Read the model definition and answer for the solid it produces. Units are mm, in the model's axes. A direction names the side the tool comes from. Coordinates: 2 decimals unless noted, no trailing zeros. Write each loop counter-clockwise with the first axis right and the second up, starting at its lowest first coordinate (ties: lowest second). Pieces come first, ordered by that corner, then holes. Notation, with made-up numbers: (-26, -23) -> (12, -23) arc R16 ccw to (12, -4) -> close; hole circle Ø9 at (-36.75, -19). An arc over 180 degrees is marked (long way). Answer as a JSON object with one key per item and string values. Group by question number.
(1) For a pull along Y with two mould halves and no side action, classify faces 3 (the face through (0, 23, 0)), 4 (the face through (2, 27, 1)), 5 (the face through (0, 0, 0)), 6 (the face through (-2, 28, 0)) as +Y half, -Y half, draft (parallel to the pull), parting line (faces both ways), or undercut.
(2) Find section D-D (z = -1.25). Give the vertices of the cut face in (x, y).
(3) Find section B-B (y = 27). Give the vertices of the cut face in (x, z).
(4) Find section C-C (x = -2.25). Give the vertices of the cut face in (y, z), then the cut area to 3 significant figures.
(5) Which of the six approach directions +Z, -Z, +X, -X, +Y, -Y give full straight-line access (tool end or side, diameter ignored) to faces 1 (the face through (-1.3, 25.8, 0)), 2 (the face through (0, 15, -3))?
(6) Straight lines are drawn through the part: L1, parallel to Y at x = -2.1, z = 0; L2, parallel to Y at x = -1, z = -0.5; L3, parallel to Z at x = -2, y = 27. For each, find the intervals that lie inside material, in ascending order.
(7) Find section A-A (z = 0). Give the vertices of the cut face in (x, y), then the cut area to 3 significant figures.
(8) Flat-ended cylindrical pins translate along their axes: P1, Ø1, axis at y = 17, z = -1, coming from the +X side; P2, Ø1.5, axis at x = -1, y = 13, coming from the +Z side; P3, Ø1.5, axis at y = 13, z = 2, coming from the -X side. Find the tip coordinate at first contact, or state that the pin passes through.
from build123d import *

# Parameters (mm, degrees)
SKETCH_1_R               = 3
EXTRUDE_1_DEPTH          = 30
SKETCH_2_W               = 2.6
SKETCH_2_H               = 6.217658974
CUT_EXTRUDE_1_DEPTH      = 7
CUT_EXTRUDE_3_DEPTH      = 31.454720488
CUT_EXTRUDE_3_DEPTH_BACK = 31.454720488
SKETCH_3_R               = 1


with BuildPart() as part:
    # 草图1 → 凸台-拉伸1 (new body)
    with BuildSketch(Plane(origin=(0, 0, 0), x_dir=(1, 0, 0), z_dir=(0, 1, 0))):
        with Locations(Location((0, 0, 0), (0, 0, 270))):
            Circle(SKETCH_1_R)
    extrude(amount=EXTRUDE_1_DEPTH)

    # 草图2 → 切除-拉伸1 (cut)
    with BuildSketch(Plane(origin=(0, 30, 0), x_dir=(1, 0, 0), z_dir=(0, 1, 0))):
        Rectangle(SKETCH_2_W, SKETCH_2_H)
    extrude(amount=-CUT_EXTRUDE_1_DEPTH, mode=Mode.SUBTRACT)

    # 草图3 → 切除-拉伸3 (cut, two sides: drawn at the far end of the back side and taken through both)
    with BuildSketch(Plane.ZY.offset(-1.3).offset(-CUT_EXTRUDE_3_DEPTH_BACK)):
        with Locations((0, 27)):
            Circle(SKETCH_3_R)
    extrude(amount=CUT_EXTRUDE_3_DEPTH + CUT_EXTRUDE_3_DEPTH_BACK, mode=Mode.SUBTRACT)


solid = part.part
Results below:
{
 "1": {"face 3": "+Y half", "face 4": "undercut", "face 5": "-Y half", "face 6": "undercut"},
 "2": {"outline": "(-2.73, 0) -> (2.73, 0) -> (2.73, 30) -> (1.3, 30) -> (1.3, 23) -> (-1.3, 23) -> (-1.3, 30) -> (-2.73, 30) -> close"},
 "3": {"outline": "(-2.83, -1) arc R3 ccw to (-1.3, -2.7) -> (-1.3, -1) -> close; (-2.83, 1) -> (-1.3, 1) -> (-1.3, 2.7) arc R3 ccw to start; (1.3, -2.7) arc R3 ccw to (2.83, -1) -> (1.3, -1) -> close; (1.3, 1) -> (2.83, 1) arc R3 ccw to (1.3, 2.7) -> close"},
 "4": {"outline": "(0, -1.98) -> (30, -1.98) -> (30, 1.98) -> (0, 1.98) -> close; hole circle Ø2 at (27, 0)", "area": "116 mm2"},
 "5": {"face 1": "+Z, -Z, +Y", "face 2": "+Y, -Y"},
 "6": {"L1": "y = 0 to 26, 28 to 30", "L2": "y = 0 to 23", "L3": "z = -2.24 to -1, 1 to 2.24"},
 "7": {"outline": "(-3, 0) -> (3, 0) -> (3, 26) -> (1.3, 26) -> (1.3, 23) -> (-1.3, 23) -> (-1.3, 26) -> (-3, 26) -> close; (-3, 28) -> (-1.3, 28) -> (-1.3, 30) -> (-3, 30) -> close; (1.3, 28) -> (3, 28) -> (3, 30) -> (1.3, 30) -> close", "area": "155 mm2"},
 "8": {"P1": "stops at x = 2.96", "P2": "stops at z = 2.99", "P3": "stops at x = -2.73"}
}
